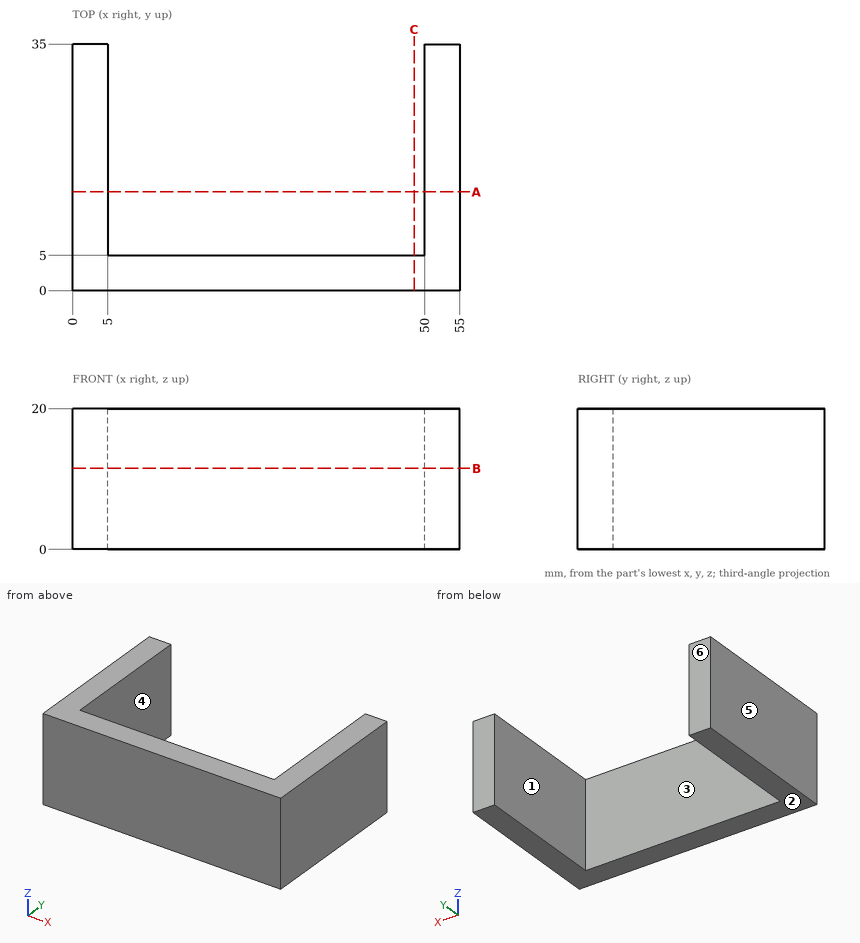
Design review of the part shown in the three views and the two pictorial views. Dimensions are in mm from the part's minimum x, y and z. A direction names the side the tool comes from. Coordinates: 2 decimals unless noted, no trailing zeros. Loops run counter-clockwise (first coordinate to the right, second up) from the corner with the lowest first, then second, coordinate; pieces in that order, holes last. Notation, with made-up numbers: M 11.25,-2 L 37.25,-2 A15 cw 37.25,7 Z; hole C 81.25,9 d8. An arc over 180 degrees is marked long. One line per question, with ' | ' between items.
(1) For pin 1 Ø6 at (x, z) = (22.5, 5.5) entering from +Y; pin 2 Ø10 at (x, y) = (14, 17.5) entering from +Z, all flat-tipped, find the tip position at first contact; note any pin that passes through.
Filled in:
pin 1: stops at y = 5 | pin 2: passes through
(2) Wall thickness on probe 1 along X at (y, z) = (10, 18); probe 2 along Y at (x, z) = (21, 15.25): over which ranges is each line inside the solid? List them lowest first.
Filled in:
probe 1: x = 0 to 5, 50 to 55 | probe 2: y = 0 to 5
(3) We need section C-C (x = 48.5). Give the boundary of the cut face in (y, z), and give its area (3 significant figures).
Filled in:
outline: M 0,0 L 5,0 L 5,20 L 0,20 Z | area: 100 mm^2
(4) We need section A-A (y = 14). Give the boundary of the cut face in (x, z).
Filled in:
outline: M 0,0 L 5,0 L 5,20 L 0,20 Z; M 50,0 L 55,0 L 55,20 L 50,20 Z
(5) Machinability: for the marked faces 1 and 2, which of the approach directions +Z, -Z, +X, -X, +Y, -Y give a long, thin tool a straight path to every point of the face, cutting with its end or side? Answer none if there is none.
Filled in:
face 1: +Z, -Z, +Y | face 2: -Z, +X, -X, +Y, -Y
(6) We need section B-B (z = 11.5). Give the boundary of the cut face in (x, y), and give its area (3 significant figures).
Filled in:
outline: M 0,0 L 55,0 L 55,35 L 50,35 L 50,5 L 5,5 L 5,35 L 0,35 Z | area: 575 mm^2
(7) Draft analysis for pull direction X (two halves, no side actions). For the marked faces 3, 4, 5 and 6, state which applies: released by +X, released by -X, zero draft, split by the parting line, or undercut.
Filled in:
face 3: undercut | face 4: undercut | face 5: released by -X | face 6: zero draft
